Source: three-view drawing plus pictorial views. Frame: mm from the lowest corner of the part. Coordinates: 2 decimals unless noted, no trailing zeros. Write each loop counter-clockwise with the first axis right and the second up, starting at its lowest first coordinate (ties: lowest second). Pieces come first, ordered by that corner, then holes. Notation, with made-up numbers: (29, 44.25) -> (74, 44.25) arc R35 cw to (74, 77.25) -> close; hole circle Ø5 at (73.5, 36.25). An arc over 180 degrees is marked (long way). One line per item, written item: value.
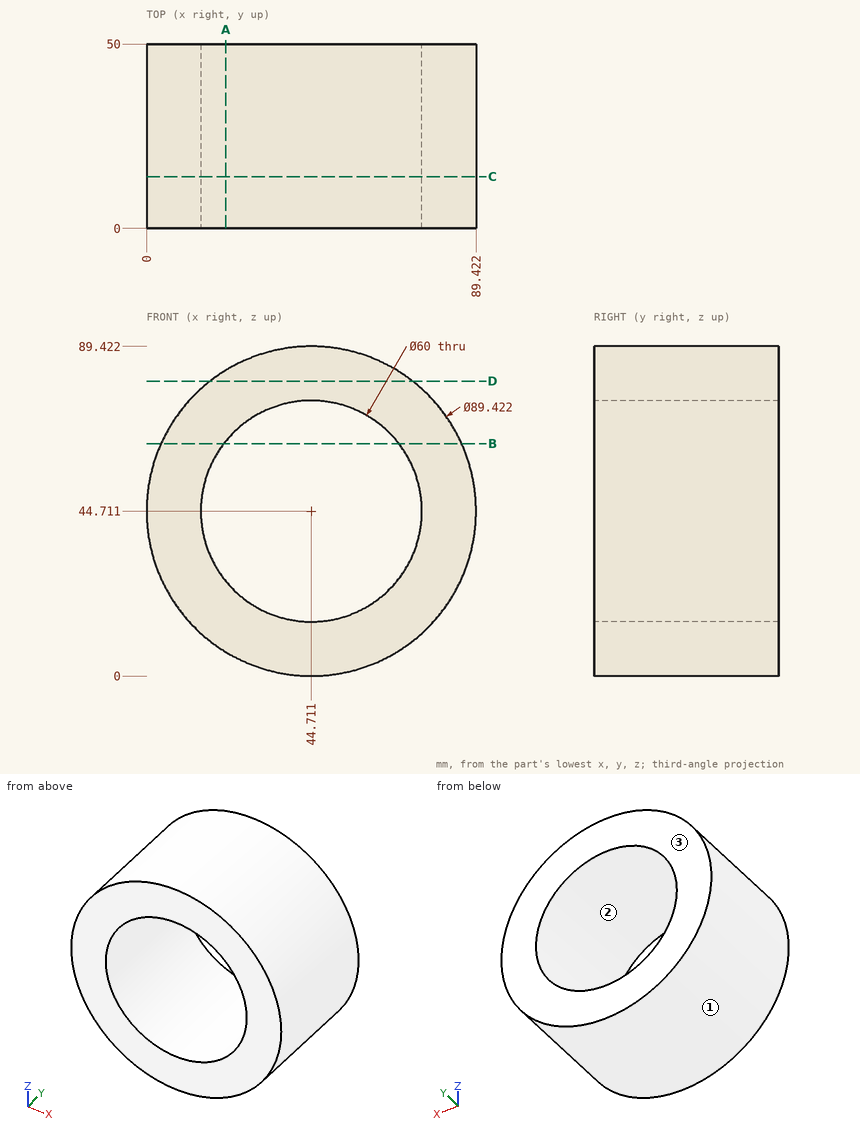
(1) Section D-D (z = 80). Return the cut outline in (x, y), then the cut area to 3 significant figures.
Responses:
outline: (17.26, 0) -> (72.17, 0) -> (72.17, 50) -> (17.26, 50) -> close
area: 2,750 mm2
(2) First-contact query: pin 1 (2 mm diameter, centred on x = 23, y = 24.5, fed in from +Z); pin 2 (4 mm diameter, centred on x = 18, y = 9, fed in from -Z); pin 3 (2 mm diameter, centred on y = 22.5, z = 26, fed in from +X). Flat tips, straight axial feed; report the tip coordinate or a pass-through.
Responses:
pin 1: stops at z = 84.34
pin 2: stops at z = 7.45
pin 3: stops at x = 85.76
(3) Section B-B (z = 63). Return the cut outline in (x, y).
Responses:
outline: (3.91, 0) -> (20.93, 0) -> (20.93, 50) -> (3.91, 50) -> close; (68.49, 0) -> (85.51, 0) -> (85.51, 50) -> (68.49, 50) -> close
(4) Section C-C (y = 14). Return the cut outline in (x, z), then the cut area to 3 significant figures.
Responses:
outline: circle Ø89.42 at (44.71, 44.71); hole circle Ø60 at (44.71, 44.71)
area: 3,450 mm2
(5) Line query: line 1 (X direction, y = 34, z = 36); line 2 (Z direction, x = 49, y = 35); line 3 (X direction, y = 29, z = 69.5). Output: solid intervals per line, ascending. Write a range as [from, to].
Responses:
line 1: x = [0.86, 16], [73.42, 88.57]
line 2: z = [0.21, 15.02], [74.4, 89.22]
line 3: x = [7.5, 27.81], [61.61, 81.92]
(6) Pull-direction query (X, two-part tool) for the marked faces 1, 2 and 3; classes: released by +X, released by -X, zero draft, split by the parting line, or undercut.
Responses:
face 1: split by the parting line
face 2: undercut
face 3: zero draft
(7) Section A-A (x = 21.5). Return the cut outline in (y, z), then the cut area to 3 significant figures.
Responses:
outline: (0, 6.5) -> (50, 6.5) -> (50, 25.7) -> (0, 25.7) -> close; (0, 63.72) -> (50, 63.72) -> (50, 82.93) -> (0, 82.93) -> close
area: 1,920 mm2
